from build123d import *

# Parameters (mm, degrees)
SKETCH1_R            = 6
BOSS_EXTRUDE1_DEPTH  = 25
M6_CLEARANCE_HOLE1_D = 6.6
CHAMFER1_SIZE        = 0.2


with BuildPart() as part:
    # Sketch1 → Boss-Extrude1 (new body)
    with BuildSketch(Plane(origin=(0, 0, 0), x_dir=(1, 0, 0), z_dir=(0, 1, 0))):
        Circle(SKETCH1_R)
    extrude(amount=BOSS_EXTRUDE1_DEPTH)

    # M6 Clearance Hole1 (through all)
    with Locations(Plane(origin=(0, 25, 0), x_dir=(1, 0, 0), z_dir=(0, 1, 0))):
        with Locations((0, 0)):
            Hole(M6_CLEARANCE_HOLE1_D / 2)

    # Chamfer1
    chamfer1_edges = [part.edges().sort_by_distance(p)[0] for p in [
        (-6, 0, 0),
        (-6, 25, 0),
        (3.3, 25, 0),
        (3.3, 0, 0),
    ]]
    chamfer(chamfer1_edges, length=CHAMFER1_SIZE)


solid = part.part
Geometry: final body of the model. Coordinates: model frame, mm. Coordinates: 2 decimals unless noted, no trailing zeros. Order: outer loops, then holes, each group sorted by start corner. A loop starts at its lowest first (then second) coordinate and runs counter-clockwise, first axis right, second up.
1) Section B-B (z = 0). Return loops of the section in (x, y).
Result sheet:
outline: (-6, 0.2) - (-5.8, 0) - (-3.5, 0) - (-3.3, 0.2) - (-3.3, 24.8) - (-3.5, 25) - (-5.8, 25) - (-6, 24.8) - close; (3.3, 0.2) - (3.5, 0) - (5.8, 0) - (6, 0.2) - (6, 24.8) - (5.8, 25) - (3.5, 25) - (3.3, 24.8) - close
2) Section C-C (y = 6.5). Return loops of the section in (x, z), then the cut area to 3 significant figures.
Result sheet:
outline: circle Ø12 at (0, 0); hole circle Ø6.6 at (0, 0)
area: 78.9 mm2
3) Section A-A (x = 0). Return loops of the section in (y, z).
Result sheet:
outline: (0, -5.8) - (0.2, -6) - (24.8, -6) - (25, -5.8) - (25, -3.5) - (24.8, -3.3) - (0.2, -3.3) - (0, -3.5) - close; (0, 3.5) - (0.2, 3.3) - (24.8, 3.3) - (25, 3.5) - (25, 5.8) - (24.8, 6) - (0.2, 6) - (0, 5.8) - close
4) Ray query, probe 1 along Z at (x, y) = (0, 19.25); probe 2 along X at (y, z) = (7, 2.25). Return the intervals inside material, ascending.
Result sheet:
probe 1: z = -6 to -3.3, 3.3 to 6
probe 2: x = -5.56 to -2.41, 2.41 to 5.56
5) First-contact query: P1, Ø2, axis at x = -2.5, y = 12.5, coming from the -Z side; P2, Ø3, axis at x = 4, y = 19, coming from the +Z side; P3, Ø1, axis at y = 9.5, z = -4, coming from the +X side. Flat tips, straight axial feed; report the tip coordinate or a pass-through.
Result sheet:
P1: stops at z = -5.81
P2: stops at z = 5.45
P3: stops at x = 4.87
